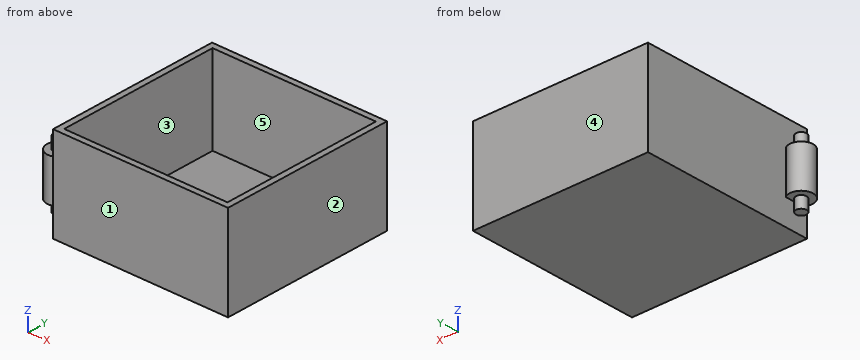
```python
from build123d import *

# Parameters (mm, degrees)
F0_W     = 75
F0_H     = 75
F1_DEPTH = 40
F2_T     = -2.5
F5_DEPTH = 9
F7_R     = 2.25
F8_DEPTH = 5
F6_R     = 2.25
F9_DEPTH = 5


with BuildPart() as f1:
    # F0 (on Top) → F1 (new body)
    with BuildSketch(Plane.XY):
        with Locations((37.5, 37.5)):
            Rectangle(F0_W, F0_H)
    extrude(amount=F1_DEPTH)

    # F2
    f2_openings = [f1.faces().sort_by_distance(p)[0] for p in [
        (37.5, 37.5, 40),
    ]]
    offset(amount=F2_T, openings=f2_openings)

    # F4 (on offset) → F5 (join, symmetric)
    with BuildSketch(Plane(origin=(0, 0, 20), x_dir=(1, 0, 0), z_dir=(0, 0, -1))):
        with BuildLine():
            Line((0, -10), (0, -2))
            ThreePointArc((0, -2), (-8, -6), (0, -10))
        make_face()
    extrude(amount=F5_DEPTH, both=True)

    # F7 (on face) → F8 (join)
    with BuildSketch(Plane(origin=(0, 0, 11), x_dir=(1, 0, 0), z_dir=(0, 0, -1))):
        with Locations((-3, -6)):
            Circle(F7_R)
    extrude(amount=F8_DEPTH)

    # F6 (on face) → F9 (join)
    with BuildSketch(Plane.XY.offset(29)):
        with Locations((-3, 6)):
            Circle(F6_R)
    extrude(amount=F9_DEPTH)


solid = f1.part
```
Check sheet for the modelled part. Datum: model origin and axes. Units: mm. Face numbers are marked on the shaded views. A direction names the side the tool comes from. Round coordinates to 2 decimals unless told otherwise and drop trailing zeros. Order: outer loops, then holes, each group sorted by start corner. A loop starts at its lowest first (then second) coordinate and runs counter-clockwise, first axis right, second up. Notation, with made-up numbers: M 22.25,-21.75 L 60.25,-21.75 A4 ccw 60.25,-16.75 Z; hole C 76,32.5 d8. An arc over 180 degrees is marked long. Answer in a Markdown table with one row per item.
(1) Section check C-C on x = 55.5. Record the boundary of the cut face in (y, z).
Findings:
| item | result |
|---|---|
| outline | M 0,0 L 75,0 L 75,40 L 72.5,40 L 72.5,2.5 L 2.5,2.5 L 2.5,40 L 0,40 Z |
(2) Section check A-A on y = 6. Record the boundary of the cut face in (x, z), plus the area to 3 significant figures.
Findings:
| item | result |
|---|---|
| outline | M -8,11 L -5.25,11 L -5.25,6 L -0.75,6 L -0.75,11 L 0,11 L 0,0 L 75,0 L 75,40 L 72.5,40 L 72.5,2.5 L 2.5,2.5 L 2.5,40 L 0,40 L 0,29 L -0.75,29 L -0.75,34 L -5.25,34 L -5.25,29 L -8,29 Z |
| area | 564 mm^2 |
(3) Gauge pin test, flat ends, axial feed: pin 1 (3.5 mm diameter, centred on x = -4, y = 6.5, fed in from +Z); pin 2 (1.5 mm diameter, centred on x = 19.5, y = 17.5, fed in from +Z); pin 3 (5 mm diameter, centred on y = 48, z = 17, fed in from -X). Record the tip position at first contact, or that the pin passes through.
Findings:
| item | result |
|---|---|
| pin 1 | stops at z = 34 |
| pin 2 | stops at z = 2.5 |
| pin 3 | stops at x = 0 |
(4) Draft check along X on the marked faces 1, 2 and 3. Enter one of: +X half, -X half, draft (parallel to the pull), parting line (faces both ways), or undercut.
Findings:
| item | result |
|---|---|
| face 1 | draft |
| face 2 | +X half |
| face 3 | undercut |
(5) Material ranges on line 1 along X through (y, z) = (49.5, 34.5); line 2 along Z through (x, y) = (39.5, 66.5), recorded low to high. Write a range as from..to.
Findings:
| item | result |
|---|---|
| line 1 | x = 0..2.5, 72.5..75 |
| line 2 | z = 0..2.5 |
(6) Section check B-B on z = 14. Record the boundary of the cut face in (x, y), plus the area to 3 significant figures.
Findings:
| item | result |
|---|---|
| outline | M 0,0 L 75,0 L 75,75 L 0,75 L 0,10 A5 ccw long 0,2 Z; hole M 2.5,2.5 L 72.5,2.5 L 72.5,72.5 L 2.5,72.5 Z |
| area | 792 mm^2 |
(7) Set-up check for the marked faces 4 and 5: record each of +Z, -Z, +X, -X, +Y, -Y from which the full face is reachable in a straight line by a thin tool's end or side.
Findings:
| item | result |
|---|---|
| face 4 | +Z, -Z, +X, -X, +Y |
| face 5 | +Z |
